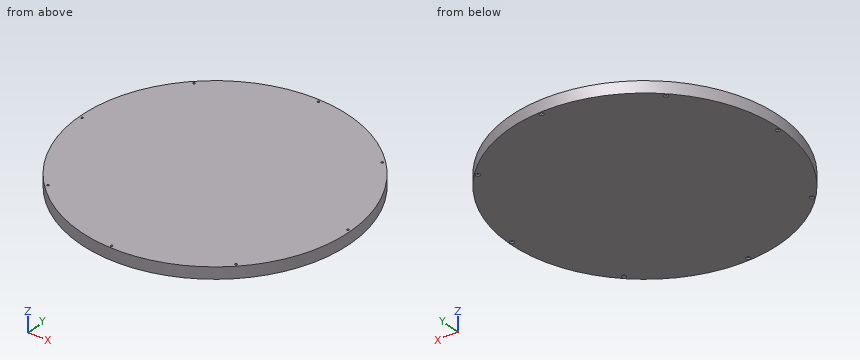
```python
from build123d import *

# Parameters (mm, degrees)
SKETCH1_R                                       = 140
BOSS_EXTRUDE1_DEPTH                             = 12
CSK_FOR_M2_FLAT_HEAD_MACHINE_SCREW1_D           = 2.2
CSK_FOR_M2_FLAT_HEAD_MACHINE_SCREW1_CSINK_D     = 4.4
CSK_FOR_M2_FLAT_HEAD_MACHINE_SCREW1_CSINK_ANGLE = 90


with BuildPart() as part:
    # Sketch1 → Boss-Extrude1 (new body)
    with BuildSketch(Plane.XY):
        Circle(SKETCH1_R)
    extrude(amount=BOSS_EXTRUDE1_DEPTH)

    # CSK for M2 Flat Head Machine Screw1 (through all)
    with Locations(Plane(origin=(0, 0, 0), x_dir=(-1, 0, 0), z_dir=(0, 0, -1))):
        with Locations((0, 137), (137, 0), (0, -137), (-137, 0), (-96.874, 96.874), (96.874, 96.874), (96.874, -96.874), (-96.874, -96.874)):
            CounterSinkHole(CSK_FOR_M2_FLAT_HEAD_MACHINE_SCREW1_D / 2, CSK_FOR_M2_FLAT_HEAD_MACHINE_SCREW1_CSINK_D / 2, counter_sink_angle=CSK_FOR_M2_FLAT_HEAD_MACHINE_SCREW1_CSINK_ANGLE)


solid = part.part
```
Input: part model. Units: mm. Frame: model coordinates. Round coordinates to 2 decimals unless told otherwise and drop trailing zeros. Loops run counter-clockwise (first coordinate to the right, second up) from the corner with the lowest first, then second, coordinate; pieces in that order, holes last. Notation, with made-up numbers: M -31.5,72 L 25.5,72 A18 ccw 25.5,85 Z; hole C 73,-24.5 d11. An arc over 180 degrees is marked long. Answer in a Markdown table with one row per item. Add a question column.
1. Ray query, probe 1 along Y at (x, z) = (0, 4.75); probe 2 along X at (y, z) = (97.5, 2.5); probe 3 along Y at (x, z) = (96, 2.25). Return the intervals inside material, ascending.
2. Contact query for flat-ended pins moving along their axis: pin 1 (2.5 mm diameter, centred on x = 0, y = 137, fed in from -Z); pin 2 (1.8 mm diameter, centred on x = -96.874, y = -96.874, fed in from +Z); pin 3 (3.5 mm diameter, centred on x = -96.874, y = 96.874, fed in from +Z); pin 4 (3 mm diameter, centred on x = 50, z = 6.5, fed in from -Y). Output: stop coordinate, or through.
3. Section C-C (y = -104). Output: boundary loops of the cut face in (x, z), and give its area (3 significant figures).
4. Section B-B (x = 86.5). Output: boundary loops of the cut face in (y, z), and give its area (3 significant figures).
5. Section A-A (z = 3). Give the number of separate pieces and of enclosed holes in the cut face, and give its area (3 significant figures).
Values follow:
| question | item | result |
|---|---|---|
| 1 | probe 1 | -140 to -138.1, -135.9 to 135.9, 138.1 to 140 |
| 1 | probe 2 | -100.47 to -97.78, -95.97 to 95.97, 97.78 to 100.47 |
| 1 | probe 3 | -101.9 to -97.54, -96.21 to 96.21, 97.54 to 101.9 |
| 2 | pin 1 | z = 0.95 |
| 2 | pin 2 | through |
| 2 | pin 3 | z = 12 |
| 2 | pin 4 | y = -131.33 |
| 3 | outline | M -93.72,0 L 93.72,0 L 93.72,12 L -93.72,12 Z |
| 3 | area | 2,250 mm^2 |
| 4 | outline | M -110.08,0 L 110.08,0 L 110.08,12 L -110.08,12 Z |
| 4 | area | 2,640 mm^2 |
| 5 | separate pieces | 1 |
| 5 | enclosed holes | 8 |
| 5 | area | 61,500 mm^2 |
